```python
from build123d import *

# Parameters (mm, degrees)
BOSS_EXTRUDE1_DEPTH = 6
FILLET1_R           = 0.5
SKETCH2_R           = 2
CUT_EXTRUDE1_DEPTH  = 12.916375288


with BuildPart() as part:
    # Sketch1 → Boss-Extrude1 (new body)
    with BuildSketch(Plane.XY):
        Polygon((0, 0), (6, 0), (9, 3), (9, 4), (6, 4), (6, 5), (0, 5), (0, 4), (-3, 4), (-3, 3), align=None)
    extrude(amount=BOSS_EXTRUDE1_DEPTH)

    # Fillet1
    fillet1_edges = [part.edges().sort_by_distance(p)[0] for p in [
        (7.5, 1.5, 6),
        (0, 4.5, 0),
        (3, 5, 0),
        (6, 4.5, 0),
        (7.5, 4, 0),
        (9, 3.5, 0),
        (7.5, 1.5, 0),
        (3, 0, 0),
        (-1.5, 1.5, 0),
        (9, 3.5, 6),
        (7.5, 4, 6),
        (-3, 4, 3),
        (0, 5, 3),
        (6, 5, 3),
        (9, 4, 3),
        (6, 0, 3),
        (0, 0, 3),
        (6, 4.5, 6),
        (3, 5, 6),
        (0, 4.5, 6),
        (-1.5, 4, 6),
        (-3, 3.5, 6),
        (-1.5, 1.5, 6),
        (3, 0, 6),
        (-3, 3.5, 0),
        (-1.5, 4, 0),
    ]]
    fillet(fillet1_edges, radius=FILLET1_R)

    # Sketch2 → Cut-Extrude1 (cut, through all)
    with BuildSketch(Plane(origin=(0, 5, 0), x_dir=(1, 0, 0), z_dir=(0, 1, 0))):
        with Locations(Location((3, -3, 0), (0, 0, 270))):
            Circle(SKETCH2_R)
    extrude(amount=-CUT_EXTRUDE1_DEPTH, mode=Mode.SUBTRACT)


solid = part.part
```
Model file for the job. Use its own axes, mm. A direction names the side the tool comes from. Coordinates: 2 decimals unless noted, no trailing zeros. Loops run counter-clockwise (first coordinate to the right, second up) from the corner with the lowest first, then second, coordinate; pieces in that order, holes last. Notation, with made-up numbers: (75, 72.5) -> (98, 72.5) arc R16 cw to (98, 96.5) -> close; hole circle Ø3 at (-13.5, 40.5). An arc over 180 degrees is marked (long way). Answer as a JSON object with one key per item and string values.
Q1. Pull direction Z, two halves, no side cores. Call faces 3 (the flat face through (-1, 4, 3)), 4 (the cylindrical face through (-1.45, 1.65, 5.85)), 5 (the cylindrical face through (1, 3, 3)): released by +Z, released by -Z, zero draft, split by the parting line, or undercut.
Report:
{"face 3": "zero draft", "face 4": "released by +Z", "face 5": "undercut"}
Q2. 3-axis set-ups, long thin cutter, end or side, ignore diameter. For faces 1 (the flat face through (5, 5, 2)), 2 (the flat face through (7, 4, 3)): which of +Z, -Z, +X, -X, +Y, -Y reach the whole face in a straight line?
Report:
{"face 1": "+Z, -Z, +X, -X, +Y", "face 2": "+Z, -Z, +X, +Y"}
Q3. Cut at B-B (x = 3). List the corners of the cut face in (y, z), and give its area (3 significant figures).
Report:
{"outline": "(0, 0.5) arc R0.5 ccw to (0.5, 0) -> (4.5, 0) arc R0.5 ccw to (5, 0.5) -> (5, 1) -> (0, 1) -> close; (0, 5) -> (5, 5) -> (5, 5.5) arc R0.5 ccw to (4.5, 6) -> (0.5, 6) arc R0.5 ccw to (0, 5.5) -> close", "area": "9.79 mm2"}
Q4. Cut at A-A (z = 3). List the corners of the cut face in (x, y), and give its area (3 significant figures).
Report:
{"outline": "(-3, 3) -> (-0.15, 0.15) arc R0.5 ccw to (0.21, 0) -> (1, 0) -> (1, 5) -> (0.5, 5) arc R0.5 ccw to (0, 4.5) -> (0, 4) -> (-2.5, 4) arc R0.5 ccw to (-3, 3.5) -> close; (5, 0) -> (5.79, 0) arc R0.5 ccw to (6.15, 0.15) -> (9, 3) -> (9, 3.5) arc R0.5 ccw to (8.5, 4) -> (6, 4) -> (6, 4.5) arc R0.5 ccw to (5.5, 5) -> (5, 5) -> close", "area": "24.8 mm2"}
Q5. Probe probe 1 along Z at (x, y) = (3.75, 1); probe 2 along X at (y, z) = (0.85, 1.25); probe 3 along X at (y, z) = (1.95, 3). List the from-to ranges inside material, lowest first.
Report:
{"probe 1": "z = 0 to 1.15, 4.85 to 6", "probe 2": "x = -0.85 to 2.03, 3.97 to 6.85", "probe 3": "x = -1.95 to 1, 5 to 7.95"}
Q6. Cut at C-C (z = 1.25). List the corners of the cut face in (x, y).
Report:
{"outline": "(-3, 3) -> (-0.15, 0.15) arc R0.5 ccw to (0.21, 0) -> (2.03, 0) -> (2.03, 5) -> (0.5, 5) arc R0.5 ccw to (0, 4.5) -> (0, 4) -> (-2.5, 4) arc R0.5 ccw to (-3, 3.5) -> close; (3.97, 0) -> (5.79, 0) arc R0.5 ccw to (6.15, 0.15) -> (9, 3) -> (9, 3.5) arc R0.5 ccw to (8.5, 4) -> (6, 4) -> (6, 4.5) arc R0.5 ccw to (5.5, 5) -> (3.97, 5) -> close"}
Q7. Cut at D-D (z = 5.75). List the corners of the cut face in (x, y).
Report:
{"outline": "(-2.93, 3.03) -> (-0.1, 0.19) arc R0.43 ccw to (0.21, 0.07) -> (5.79, 0.07) arc R0.43 ccw to (6.1, 0.19) -> (8.93, 3.03) -> (8.93, 3.5) arc R0.43 ccw to (8.5, 3.93) -> (5.93, 3.93) -> (5.93, 4.5) arc R0.43 ccw to (5.5, 4.93) -> (0.5, 4.93) arc R0.43 ccw to (0.07, 4.5) -> (0.07, 3.93) -> (-2.5, 3.93) arc R0.43 ccw to (-2.93, 3.5) -> close"}
Q8. Flat gauge pins, fed straight in: P1, Ø0.6, axis at y = 4, z = 2, coming from the +X side; P2, Ø1.2, axis at x = 7.5, z = 4, coming from the +Y side. Where does each tip first touch, or does it go through?
Report:
{"P1": "stops at x = 8.96", "P2": "stops at y = 4"}
